```python
from build123d import *

# Parameters (mm, degrees)
SKETCH1_R           = 7.5
BOSS_EXTRUDE1_DEPTH = 5
SKETCH2_R           = 3.5
BOSS_EXTRUDE2_DEPTH = 13
CHAMFER1_SIZE       = 0.5
BOSS_EXTRUDE3_DEPTH = 2
SKETCH4_R           = 1.5
BOSS_EXTRUDE4_DEPTH = 5


with BuildPart() as part:
    # Sketch1 → Boss-Extrude1 (new body)
    with BuildSketch(Plane.XY):
        Circle(SKETCH1_R)
    extrude(amount=BOSS_EXTRUDE1_DEPTH)

    # Sketch2 → Boss-Extrude2 (add)
    with BuildSketch(Plane.XY.offset(5)):
        Circle(SKETCH2_R)
    extrude(amount=BOSS_EXTRUDE2_DEPTH)

    # Chamfer1
    chamfer1_edges = [part.edges().sort_by_distance(p)[0] for p in [
        (-3.5, 0, 18),
    ]]
    chamfer(chamfer1_edges, length=CHAMFER1_SIZE)

    # Sketch3 → Boss-Extrude3 (add)
    with BuildSketch(Plane(origin=(0, 0, 0), x_dir=(-1, 0, 0), z_dir=(0, 0, -1))):
        with BuildLine():
            Line((3, 0), (3, -30))
            ThreePointArc((3, -30), (0, -33), (-3, -30))
            Line((-3, -30), (-3, 0))
            ThreePointArc((-3, 0), (0, 3), (3, 0))
        make_face()
    extrude(amount=BOSS_EXTRUDE3_DEPTH)

    # Sketch4 → Boss-Extrude4 (add)
    with BuildSketch(Plane(origin=(0, 0, -2), x_dir=(-1, 0, 0), z_dir=(0, 0, -1))):
        with Locations((0, -30)):
            Circle(SKETCH4_R)
    extrude(amount=BOSS_EXTRUDE4_DEPTH)


solid = part.part
```
For this review, take the finished solid that the model builds, in its own axes (mm). A direction names the side the tool comes from. Round coordinates to 2 decimals unless told otherwise and drop trailing zeros. Write each loop counter-clockwise with the first axis right and the second up, starting at its lowest first coordinate (ties: lowest second). Pieces come first, ordered by that corner, then holes. Notation, with made-up numbers: (49, 81.25) - (73, 81.25) arc R14 ccw to (73, 87.25) - close; hole circle Ø8 at (-9.5, 12.5). An arc over 180 degrees is marked (long way). Answer as CSV lines item,"result". Start each with the question number.
(1) Add section C-C, the plane z = 4. State the section outline as (x, y) points, plus the area to 3 significant figures.
(2) For line 1 (Z direction, x = -2, y = -10); line 2 (Y direction, x = 0, z = -3.25); line 3 (Z direction, x = -1, y = -29), list the stretches that pass through material, from the lowest coordinate up.
(3) For pin 1 (0.6 mm diameter, centred on y = -13.5, z = -1.5, fed in from -X); pin 2 (3 mm diameter, centred on x = -1, y = -12, fed in from -Z); pin 3 (10 mm diameter, centred on y = -28, z = -1, fed in from +X); pin 4 (5 mm diameter, centred on x = 5, z = -3.5, fed in from -Y), all flat-tipped, find the tip position at first contact; note any pin that passes through.
(4) Machinability: for faces 1 (the cylindrical face through (0.195, -28.513, -4.465)), 2 (the flat face through (3.2, 1.8, 5)), 3 (the flat face through (3, -15, -1)), which of the approach directions +Z, -Z, +X, -X, +Y, -Y give a long, thin tool a straight path to every point of the face, cutting with its end or side? Answer none if there is none.
(5) Add section D-D, the plane z = 11.25. State the section outline as (x, y) points, plus the area to 3 significant figures.
(6) Add section A-A, the plane y = -6. State the section outline as (x, z) points, plus the area to 3 significant figures.
(7) Add section B-B, the plane x = 0. State the section outline as (y, z) points, plus the area to 3 significant figures.
From the geometry:
1,outline,"circle Ø15 at (0, 0)"
1,area,"177 mm²"
2,line 1,"z = -2 to 0"
2,line 2,"y = -31.5 to -28.5"
2,line 3,"z = -7 to 0"
3,pin 1,"stops at x = -3"
3,pin 2,"stops at z = -2"
3,pin 3,"stops at x = 3"
3,pin 4,"passes through"
4,face 1,"-Z"
4,face 2,"+Z"
4,face 3,"-Z, +X, +Y, -Y"
5,outline,"circle Ø7 at (0, 0)"
5,area,"38.5 mm²"
6,outline,"(-4.5, 0) - (-3, 0) - (-3, -2) - (3, -2) - (3, 0) - (4.5, 0) - (4.5, 5) - (-4.5, 5) - close"
6,area,"57.0 mm²"
7,outline,"(-33, -2) - (-31.5, -2) - (-31.5, -7) - (-28.5, -7) - (-28.5, -2) - (3, -2) - (3, 0) - (7.5, 0) - (7.5, 5) - (3.5, 5) - (3.5, 17.5) - (3, 18) - (-3, 18) - (-3.5, 17.5) - (-3.5, 5) - (-7.5, 5) - (-7.5, 0) - (-33, 0) - close"
7,area,"253 mm²"
